CAD build for the part. Positions are in the model's coordinates, mm. Round coordinates to 2 decimals unless told otherwise and drop trailing zeros. Loops run counter-clockwise (first coordinate to the right, second up) from the corner with the lowest first, then second, coordinate; pieces in that order, holes last.
Autodesk Inventor part; units mm, degrees
ref_plane "YZ Plane" through (0, 0, 0) normal (1, 0, 0) x (0, 1, 0)
ref_plane "XZ Plane" through (0, 0, 0) normal (0, 1, 0) x (-1, 0, 0)
ref_plane "XY Plane" through (0, 0, 0) normal (0, 0, 1) x (1, 0, 0)
sketch "Эскиз1" plane through (0, 0, 0) normal (0, 0, 1) x (1, 0, 0)
  line L0 (-251.3272, 12) -> (251.3272, 12)
  line L1 (251.3272, 12) -> (251.3272, 0)
  line L2 (251.3272, 0) -> (-251.3272, 0)
  line L3 (-251.3272, 0) -> (-251.3272, 12)
  point P0 (0, 0)
  point P1 (0, 0)
  dimension "d0" = 12
  dimension "d1" = 502.6544
extrude "Выдавливание1" add sketch "Эскиз1" against normal blind 2
sketch "Эскиз4" plane through (0, 0, 0) normal (0, 0, 1) x (1, 0, 0)
  arc A0 (-243.8272, 8.5) -> (-243.8272, 3.5) centre (-243.8272, 6) ccw
  line L0 (-243.8272, 8.5) -> (-239.948, 8.5)
  arc A1 (-239.948, 8.5) -> (-239.1165, 8.9444) centre (-239.948, 9.5) ccw
  arc A2 (-236.8272, 8.25) -> (-239.1165, 8.9444) centre (-238.0772, 8.25) ccw
  line L1 (-236.8272, 8.25) -> (-236.8272, 3.75)
  arc A3 (-239.1165, 3.0556) -> (-236.8272, 3.75) centre (-238.0772, 3.75) ccw
  arc A4 (-239.1165, 3.0556) -> (-239.948, 3.5) centre (-239.948, 2.5) ccw
  line L2 (-239.948, 3.5) -> (-243.8272, 3.5)
  arc A5 (217.9113, 0) -> (219.9113, 2) centre (217.9113, 2) ccw construction
  line L3 (219.9113, 2.25) -> (219.9113, 2) construction
  arc A6 (221.1613, 3.5) -> (219.9113, 2.25) centre (221.1613, 2.25) ccw construction
  line L4 (227.4618, 3.5) -> (221.1613, 3.5) construction
  arc A7 (227.4618, 3.5) -> (227.4618, 8.5) centre (229.9113, 6) ccw construction
  line L5 (221.1613, 8.5) -> (227.4618, 8.5) construction
  arc A8 (219.9113, 9.75) -> (221.1613, 8.5) centre (221.1613, 9.75) ccw construction
  line L6 (219.9113, 10) -> (219.9113, 9.75) construction
  arc A9 (219.9113, 10) -> (217.9113, 12) centre (217.9113, 10) ccw construction
  line L7 (-249.3272, 12) -> (217.9113, 12) construction
  arc A10 (-249.3272, 12) -> (-251.3272, 10) centre (-249.3272, 10) ccw construction
  line L8 (-251.3272, 2) -> (-251.3272, 10) construction
  arc A11 (-251.3272, 2) -> (-249.3272, 0) centre (-249.3272, 2) ccw construction
  line L9 (217.9113, 0) -> (-249.3272, 0) construction
  line L10 (252.5772, 8.5) -> (258.8777, 8.5)
  arc A12 (258.8777, 3.5) -> (258.8777, 8.5) centre (261.3272, 6) ccw
  line L11 (258.8777, 3.5) -> (252.5772, 3.5)
  arc A13 (252.5772, 3.5) -> (251.3272, 2.25) centre (252.5772, 2.25) ccw
  arc A14 (251.3272, 9.75) -> (252.5772, 8.5) centre (252.5772, 9.75) ccw
  line L12 (251.3272, 9.75) -> (251.3272, 2.25)
  line L13 (251.3272, 12) -> (251.3272, 0) construction
  point P0 (0, 0)
extrude "Выдавливание4" add sketch "Эскиз4" against normal up to surface (2 mm away) contours L10 A12 L11 A13 L12 A14
extrude "Выдавливание5" cut sketch "Эскиз4" against normal blind 10 contours L0 A1 A2 L1 A3 A4 L2 A0
fillet "Сопряжение2" radius 2 4 edges at (251.3272, 0, -1) (251.3272, 12, -1) (-251.3272, 0, -1) (-251.3272, 12, -1)
sketch "Эскиз2" plane through (0, 0, 0) normal (0, 0, 1) x (1, 0, 0)
  line L0 (-251.3272, 12) -> (251.3272, 12)
  line L1 (-251.3272, 0) -> (-251.3272, 12)
  line L2 (251.3272, 0) -> (-251.3272, 0)
  line L3 (251.3272, 12) -> (251.3272, 0)
  line L4 (0, 0) -> (0, 12)
properties part number "Пластина LED(New6)-развёртка"
Item 1: Cut at A-A (z = -1.25). List the corners of the cut face in (x, y).
Verdict:
outline: (-251.33, 2) arc R2 ccw to (-249.33, 0) - (249.33, 0) arc R2 ccw to (251.33, 2) - (251.33, 2.25) arc R1.25 cw to (252.58, 3.5) - (258.88, 3.5) arc R3.5 ccw (long way) to (258.88, 8.5) - (252.58, 8.5) arc R1.25 cw to (251.33, 9.75) - (251.33, 10) arc R2 ccw to (249.33, 12) - (-249.33, 12) arc R2 ccw to (-251.33, 10) - close; hole (-243.83, 3.5) - (-239.95, 3.5) arc R1 cw to (-239.12, 3.06) arc R1.25 ccw to (-236.83, 3.75) - (-236.83, 8.25) arc R1.25 ccw to (-239.12, 8.94) arc R1 cw to (-239.95, 8.5) - (-243.83, 8.5) arc R2.5 ccw to start
Item 2: Wall check: L1, parallel to X at y = 6.5, z = -1.35; L2, parallel to X at y = 1.5, z = -1.65; L3, parallel to X at y = 3, z = -0.6. Give the ranges that are in metal, low to high.
Verdict:
L1: x = -251.33 to -246.28, -236.83 to 264.79
L2: x = -251.26 to 251.26
L3: x = -251.33 to -239.08, -237.08 to 251.58, 259.52 to 263.13
Item 3: Cut at B-B (y = 6). List the corners of the cut face in (x, z), plus the area to 3 significant figures.
Verdict:
outline: (-251.33, -2) - (-246.33, -2) - (-246.33, 0) - (-251.33, 0) - close; (-236.83, -2) - (264.83, -2) - (264.83, 0) - (-236.83, 0) - close
area: 1,010 mm2
